For this review, take the finished solid that the model builds, in its own axes (mm). A direction names the side the tool comes from. Round coordinates to 2 decimals unless told otherwise and drop trailing zeros. Write each loop counter-clockwise with the first axis right and the second up, starting at its lowest first coordinate (ties: lowest second). Pieces come first, ordered by that corner, then holes. Notation, with made-up numbers: M 12,73 L 39,73 A37 ccw 39,111 Z; hole C 59,64 d8. An arc over 180 degrees is marked long. Answer in a Markdown table with one row per item.
```python
from build123d import *

# Parameters (mm, degrees)
BOSS_EXTRUDE1_DEPTH = 3
BOSS_EXTRUDE2_DEPTH = 4
SKETCH4_R           = 1.5
SKETCH4_R_2         = 2.5
CUT_EXTRUDE1_DEPTH  = 3
SKETCH5_R           = 1.5
CUT_EXTRUDE2_DEPTH  = 77.223356001
SKETCH6_W           = 35
SKETCH6_H           = 6.8
BOSS_EXTRUDE3_DEPTH = 3
FILLET1_R           = 3


with BuildPart() as part:
    # Sketch2 → Boss-Extrude1 (new body)
    with BuildSketch(Plane(origin=(0, 0, 0), x_dir=(1, 0, 0), z_dir=(0, 1, 0))):
        Polygon((-75, 4), (-75, -4), (75, -4), align=None)
        Polygon((75, 4), (75, -4), (-75, 4), align=None)
    extrude(amount=BOSS_EXTRUDE1_DEPTH)

    # Sketch3 → Boss-Extrude2 (add, symmetric)
    with BuildSketch(Plane.XY):
        Polygon((-58.9, 0), (-58.9, -10), (-43.9, -10), (-43.9, -13), (-61.9, -13), (-61.9, 0), align=None)
    boss_extrude2 = extrude(amount=BOSS_EXTRUDE2_DEPTH, both=True)

    # Sketch4 → Cut-Extrude1 (cut)
    with BuildSketch(Plane(origin=(0, 3, 0), x_dir=(1, 0, 0), z_dir=(0, 1, 0))):
        with Locations(Location((-71, 0, 0), (0, 0, 270))):
            Circle(SKETCH4_R)
        with Locations(Location((-51.5, 0, 0), (0, 0, 270))):
            Circle(SKETCH4_R_2)
    cut_extrude1 = extrude(amount=-CUT_EXTRUDE1_DEPTH, mode=Mode.SUBTRACT)

    # Sketch5 → Cut-Extrude2 (cut, through all)
    with BuildSketch(Plane(origin=(0, -10, 0), x_dir=(1, 0, 0), z_dir=(0, 1, 0))):
        with Locations(Location((-51.5, 0, 0), (0, 0, 270))):
            Circle(SKETCH5_R)
    cut_extrude2 = extrude(amount=-CUT_EXTRUDE2_DEPTH, mode=Mode.SUBTRACT)

    # Mirror1: Boss-Extrude2, Cut-Extrude1, Cut-Extrude2 across plane
    add(boss_extrude2.mirror(Plane(origin=(0, 0, 0), x_dir=(0, 0, 1), z_dir=(1, 0, 0))))
    add(cut_extrude1.mirror(Plane(origin=(0, 0, 0), x_dir=(0, 0, 1), z_dir=(1, 0, 0))), mode=Mode.SUBTRACT)
    add(cut_extrude2.mirror(Plane(origin=(0, 0, 0), x_dir=(0, 0, 1), z_dir=(1, 0, 0))), mode=Mode.SUBTRACT)

    # Sketch6 → Boss-Extrude3 (add)
    with BuildSketch(Plane(origin=(0, 0, -4), x_dir=(-1, 0, 0), z_dir=(0, 0, -1))):
        with Locations((0, -3.4)):
            Rectangle(SKETCH6_W, SKETCH6_H)
    extrude(amount=-BOSS_EXTRUDE3_DEPTH)

    # Fillet1
    fillet1_edges = [part.edges().sort_by_distance(p)[0] for p in [
        (-61.9, 0, 0),
        (-61.9, -13, 0),
        (-43.9, -13, 0),
        (-58.9, -10, 0),
        (58.9, -10, 0),
        (43.9, -13, 0),
        (61.9, -13, 0),
        (17.5, -6.8, -2.5),
        (0, 0, -1),
        (-17.5, -6.8, -2.5),
        (-75, 1.5, -4),
        (75, 1.5, -4),
        (75, 1.5, 4),
        (-75, 1.5, 4),
    ]]
    fillet(fillet1_edges, radius=FILLET1_R - 0.0001)  # a hair under: the kernel refuses the full size


solid = part.part
```
Q1. Take a section at B-B (x = 20.5). State the section outline as (y, z) points.
Found:
| item | result |
|---|---|
| outline | M 0,-4 L 3,-4 L 3,4 L 0,4 Z |
Q2. For probe 1 along X at (y, z) = (-4, -2.25); probe 2 along X at (y, z) = (2.1, 0); probe 3 along Y at (x, z) = (-49, -1.75), list the stretches that pass through material, from the lowest coordinate up.
Found:
| item | result |
|---|---|
| probe 1 | -61.9 to -58.9, -17.49 to 17.49, 58.9 to 61.9 |
| probe 2 | -75 to -72.5, -69.5 to -54, -49 to 49, 54 to 69.5, 72.5 to 75 |
| probe 3 | -13 to -10, 0 to 3 |
Q3. Mouldability with a two-part tool opening along Y and no side actions: class faces 4 (the face through (-58.04, -9.1, -0.06)), 5 (the face through (-17.5, -2, -2)), 6 (the face through (-44.76, -12.1, -0.06)) as +Y half, -Y half, draft (parallel to the pull), parting line (faces both ways), or undercut.
Found:
| item | result |
|---|---|
| face 4 | undercut |
| face 5 | draft |
| face 6 | -Y half |
Q4. Machinability: for faces 1 (the face through (-1, 0, 3)), 2 (the face through (58.9, -3, 0)), 3 (the face through (44.8, -12.14, -0.06)), which of the approach directions +Z, -Z, +X, -X, +Y, -Y give a long, thin tool a straight path to every point of the face, cutting with its end or side? Answer none if there is none.
Found:
| item | result |
|---|---|
| face 1 | +Z |
| face 2 | +Z, -Z |
| face 3 | +Z, -Z, -Y |
Q5. Insertion check: P1, Ø3.5, axis at x = -3.5, z = -2, coming from the -Y side; P2, Ø1.1, axis at x = -5, y = -5.5, coming from the +Z side; P3, Ø3, axis at x = -38, z = -1.5, coming from the -Y side; P4, Ø1.8, axis at x = 71, z = 0, coming from the +Y side. Each pin has a flat end and moves straight along its axis. Give the tip position at first contact, or say it passes through.
Found:
| item | result |
|---|---|
| P1 | y = -6.8 |
| P2 | z = -1 |
| P3 | y = 0 |
| P4 | through |
Q6. Take a section at A-A (x = 51.5). State the section outline as (y, z) points.
Found:
| item | result |
|---|---|
| outline | M -13,-4 L -10,-4 L -10,-1.5 L -13,-1.5 Z; M -13,1.5 L -10,1.5 L -10,4 L -13,4 Z; M 0,-4 L 3,-4 L 3,-2.5 L 0,-2.5 Z; M 0,2.5 L 3,2.5 L 3,4 L 0,4 Z |
